The listing builds one solid part. Answer for the finished solid, in the listing's coordinates (mm). Give positions to 0.01 mm unless a question says otherwise; leave off trailing zeros. Order: outer loops, then holes, each group sorted by start corner. A loop starts at its lowest first (then second) coordinate and runs counter-clockwise, first axis right, second up. Notation, with made-up numbers: (29, -21) - (45, -21) arc R22 cw to (45, -12) - close; hole circle Ø11 at (-37.75, -15.5). An arc over 180 degrees is marked (long way). Answer in a Markdown table with one row per item.
from build123d import *

# Parameters (mm, degrees)
BOSS_EXTRUDE1_DEPTH = 5
CUT_EXTRUDE3_DEPTH  = 5
SKETCH5_W           = 45
SKETCH5_H           = 10
CUT_EXTRUDE4_DEPTH  = 10
SKETCH6_W           = 10
SKETCH6_H           = 5
CUT_EXTRUDE5_DEPTH  = 5
SKETCH7_W           = 60
SKETCH7_H           = 5
BOSS_EXTRUDE2_DEPTH = 200
SKETCH8_W           = 10
SKETCH8_H           = 5
BOSS_EXTRUDE3_DEPTH = 5
SKETCH9_W           = 4
SKETCH9_H           = 5
CUT_EXTRUDE6_DEPTH  = 5
BOSS_EXTRUDE4_DEPTH = 5


with BuildPart() as part:
    # Sketch1 → Boss-Extrude1 (new body)
    with BuildSketch(Plane.XY):
        Polygon((0, -5), (10, -5), (10, 0), (13, 0), (13, 5), (10, 5), (10, 15), (20, 15), (20, 5), (17, 5), (17, 0), (20, 0), (20, -5), (80, -5), (80, 0), (83, 0), (83, 5), (80, 5), (80, 15), (90, 15), (90, 5), (87, 5), (87, 0), (90, 0), (90, -5), (100, -5), (100, 45), (90, 45), (90, 40), (87, 40), (87, 35), (90, 35), (90, 25), (80, 25), (80, 35), (83, 35), (83, 40), (80, 40), (80, 45), (20, 45), (20, 40), (17, 40), (17, 35), (20, 35), (20, 25), (10, 25), (10, 35), (13, 35), (13, 40), (10, 40), (10, 45), (0, 45), align=None)
    extrude(amount=-BOSS_EXTRUDE1_DEPTH)

    # Sketch4 → Cut-Extrude3 (cut)
    with BuildSketch(Plane(origin=(0, 0, -5), x_dir=(-1, 0, 0), z_dir=(0, 0, -1))):
        with BuildLine():
            Line((-60.15, 0.639479816), (-60.15, 18.639479816))
            ThreePointArc((-60.15, 18.639479816), (-58.15, 20.639479816), (-56.15, 18.639479816))
            Line((-56.15, 18.639479816), (-56.15, 0.639479816))
            ThreePointArc((-56.15, 0.639479816), (-58.15, -1.360520184), (-60.15, 0.639479816))
        make_face()
        with BuildLine():
            Line((-44.65, 0.639479816), (-44.65, 18.639479816))
            ThreePointArc((-44.65, 18.639479816), (-42.65, 20.639479816), (-40.65, 18.639479816))
            Line((-40.65, 18.639479816), (-40.65, 0.639479816))
            ThreePointArc((-40.65, 0.639479816), (-42.65, -1.360520184), (-44.65, 0.639479816))
        make_face()
    extrude(amount=-CUT_EXTRUDE3_DEPTH, mode=Mode.SUBTRACT)

    # Sketch5 → Cut-Extrude4 (cut)
    with BuildSketch(Plane(origin=(0, 0, -5), x_dir=(-1, 0, 0), z_dir=(0, 0, -1))):
        with Locations((-50, 32.5)):
            Rectangle(SKETCH5_W, SKETCH5_H)
    extrude(amount=-CUT_EXTRUDE4_DEPTH, mode=Mode.SUBTRACT)

    # Sketch6 → Cut-Extrude5 (cut)
    with BuildSketch(Plane.XY):
        with Locations((5, -2.5)):
            Rectangle(SKETCH6_W, SKETCH6_H)
        with Locations((95, -2.5)):
            Rectangle(SKETCH6_W, SKETCH6_H)
    extrude(amount=-CUT_EXTRUDE5_DEPTH, mode=Mode.SUBTRACT)

    # Sketch7 → Boss-Extrude2 (add)
    with BuildSketch(Plane.XZ.offset(5)):
        with Locations((50, -2.5)):
            Rectangle(SKETCH7_W, SKETCH7_H)
    extrude(amount=BOSS_EXTRUDE2_DEPTH)

    # Sketch8 → Boss-Extrude3 (add)
    with BuildSketch(Plane.XY):
        with Locations((50, -207.5)):
            Rectangle(SKETCH8_W, SKETCH8_H)
        with Locations((70, -207.5)):
            Rectangle(SKETCH8_W, SKETCH8_H)
    extrude(amount=-BOSS_EXTRUDE3_DEPTH)

    # Sketch9 → Cut-Extrude6 (cut)
    with BuildSketch(Plane.XY):
        Polygon((55, -200), (58, -200), (62, -200), (65, -200), (65, -190), (55, -190), align=None)
        with Locations((60, -202.5)):
            Rectangle(SKETCH9_W, SKETCH9_H)
    extrude(amount=-CUT_EXTRUDE6_DEPTH, mode=Mode.SUBTRACT)

    # Sketch10 → Boss-Extrude4 (add)
    with BuildSketch(Plane(origin=(0, 0, -5), x_dir=(-1, 0, 0), z_dir=(0, 0, -1))):
        with BuildLine():
            Line((-36, -287.5), (-32.66671961, -287.5))
            ThreePointArc((-32.66671961, -287.5), (-23.1851254, -246.733367303), (-20, -205))
            Line((-20, -205), (-36, -205))
            Line((-36, -205), (-36, -287.5))
        make_face()
    extrude(amount=-BOSS_EXTRUDE4_DEPTH)


solid = part.part
Item 1: Consider line 1 (Y direction, x = 62.5, z = -3.45); line 2 (Y direction, x = 37, z = -3.5); line 3 (Y direction, x = 88, z = -1). Determine where each line is inside the solid, lowest interval first.
Answer block:
| item | result |
|---|---|
| line 1 | -205 to -200, -190 to 27.5, 37.5 to 45 |
| line 2 | -205 to 27.5, 37.5 to 45 |
| line 3 | 0 to 5, 15 to 25, 35 to 40 |
Item 2: Find section A-A on z = -3.9. Count the separate pieces of the cut face and the enclosed holes in it, then the cut area to 3 significant figures.
Answer block:
| item | result |
|---|---|
| separate pieces | 1 |
| enclosed holes | 3 |
| area | 16,600 mm² |
Item 3: Find section C-C on y = -243. Write down the section's boundary in (x, z), then the cut area to 3 significant figures.
Answer block:
| item | result |
|---|---|
| outline | (22.64, -5) - (36, -5) - (36, 0) - (22.64, 0) - close |
| area | 66.8 mm² |
Item 4: Find section B-B on x = 94.5. Write down the section's boundary in (y, z).
Answer block:
| item | result |
|---|---|
| outline | (0, -5) - (45, -5) - (45, 0) - (0, 0) - close |
Item 5: Each of these flat-tipped pins is pushed along its axis until it touches: P1, Ø2.5, axis at x = 81, z = -3, coming from the -Y side; P2, Ø1.5, axis at y = -244, z = -4, coming from the +X side; P3, Ø1.5, axis at y = -60.5, z = -1, coming from the -X side. Where does it stop, or does it pass through?
Answer block:
| item | result |
|---|---|
| P1 | y = -205 |
| P2 | x = 36 |
| P3 | x = 20 |
